Here's how the part is built. I have some questions about the finished solid (model axes, mm). Face numbers are marked on the shaded views. A direction names the side the tool comes from. Round coordinates to 2 decimals unless told otherwise and drop trailing zeros. Loops run counter-clockwise (first coordinate to the right, second up) from the corner with the lowest first, then second, coordinate; pieces in that order, holes last. Notation, with made-up numbers: M -22.5,-34 L 4.5,-34 A27 cw 4.5,-12 Z; hole C 67,-9 d6. An arc over 180 degrees is marked long. Answer as a JSON object with one key per item and string values.
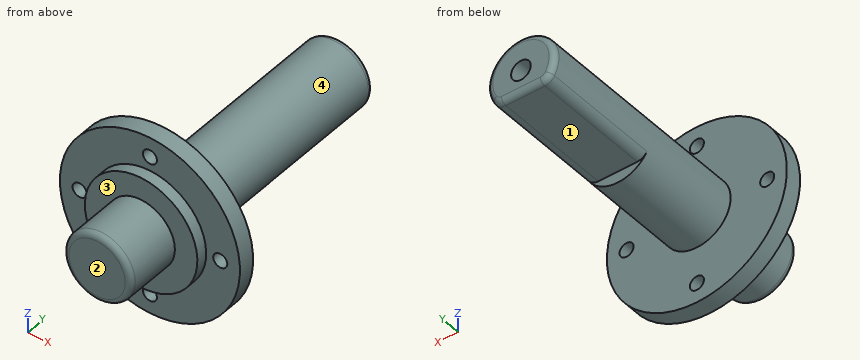
from build123d import *

# Parameters (mm, degrees)
SKETCH1_R           = 6
BOSS_EXTRUDE1_DEPTH = 10
SKETCH2_R           = 10
BOSS_EXTRUDE2_DEPTH = 2
SKETCH5_R           = 16
BOSS_EXTRUDE3_DEPTH = 3
SKETCH6_R           = 6
BOSS_EXTRUDE4_DEPTH = 40
FILLET1_R           = 1
CUT_EXTRUDE1_START  = -22
CUT_EXTRUDE1_DEPTH  = 22
FILLET2_R           = 2
FILLET3_R           = 1
SKETCH10_R          = 1.75
CUT_EXTRUDE2_DEPTH  = 20
SKETCH11_R          = 1.25
CUT_EXTRUDE3_DEPTH  = 7


with BuildPart() as part:
    # Sketch1 → Boss-Extrude1 (new body)
    with BuildSketch(Plane(origin=(0, 0, 0), x_dir=(1, 0, 0), z_dir=(0, 1, 0))):
        with Locations(Location((0, 0, 0), (0, 0, 270))):
            Circle(SKETCH1_R)
    extrude(amount=BOSS_EXTRUDE1_DEPTH)

    # Sketch2 → Boss-Extrude2 (add)
    with BuildSketch(Plane(origin=(0, 10, 0), x_dir=(1, 0, 0), z_dir=(0, 1, 0))):
        with Locations(Location((0, 0, 0), (0, 0, 270))):
            Circle(SKETCH2_R)
    extrude(amount=BOSS_EXTRUDE2_DEPTH)

    # Sketch5 → Boss-Extrude3 (add)
    with BuildSketch(Plane(origin=(0, 12, 0), x_dir=(1, 0, 0), z_dir=(0, 1, 0))):
        with Locations(Location((0, 0, 0), (0, 0, 270))):
            Circle(SKETCH5_R)
    extrude(amount=BOSS_EXTRUDE3_DEPTH)

    # Sketch6 → Boss-Extrude4 (add)
    with BuildSketch(Plane(origin=(0, 15, 0), x_dir=(1, 0, 0), z_dir=(0, 1, 0))):
        with Locations(Location((0, 0, 0), (0, 0, 270))):
            Circle(SKETCH6_R)
    extrude(amount=BOSS_EXTRUDE4_DEPTH)

    # Fillet1
    fillet1_edges = [part.edges().sort_by_distance(p)[0] for p in [
        (0, 0, -6),
    ]]
    fillet(fillet1_edges, radius=FILLET1_R)

    # Sketch7 → Cut-Extrude1 (cut)
    with BuildSketch(Plane(origin=(0, 55, 0), x_dir=(1, 0, 0), z_dir=(0, 1, 0)).offset(CUT_EXTRUDE1_START)):
        with BuildLine():
            Line((-4.472135955, 4), (4.472135955, 4))
            ThreePointArc((4.472135955, 4), (0, 6), (-4.472135955, 4))
        make_face()
    extrude(amount=CUT_EXTRUDE1_DEPTH, mode=Mode.SUBTRACT)

    # Fillet2
    fillet2_edges = [part.edges().sort_by_distance(p)[0] for p in [
        (-4.472135955, 44, -4),
        (4.472135955, 44, -4),
    ]]
    fillet(fillet2_edges, radius=FILLET2_R)

    # Fillet3
    fillet3_edges = [part.edges().sort_by_distance(p)[0] for p in [
        (5.196152423, 55, 3),
        (0, 55, -4),
        (-4.464101615, 55, -3.732050808),
        (4.464101615, 55, -3.732050808),
    ]]
    fillet(fillet3_edges, radius=FILLET3_R)

    # Sketch10 → Cut-Extrude2 (cut)
    with BuildSketch(Plane(origin=(0, 55, 0), x_dir=(1, 0, 0), z_dir=(0, 1, 0))):
        with Locations(Location((0, 0, 0), (0, 0, 270))):
            Circle(SKETCH10_R)
    extrude(amount=-CUT_EXTRUDE2_DEPTH, mode=Mode.SUBTRACT)

    # Sketch11 → Cut-Extrude3 (cut)
    with BuildSketch(Plane(origin=(0, 15, 0), x_dir=(1, 0, 0), z_dir=(0, 1, 0))):
        with Locations(Location((0, 12.5, 0), (0, 0, 270))):
            Circle(SKETCH11_R)
        with Locations(Location((12.5, 0, 0), (0, 0, 270))):
            Circle(SKETCH11_R)
        with Locations(Location((0, -12.5, 0), (0, 0, 270))):
            Circle(SKETCH11_R)
        with Locations(Location((-12.5, 0, 0), (0, 0, 270))):
            Circle(SKETCH11_R)
    extrude(amount=-CUT_EXTRUDE3_DEPTH, mode=Mode.SUBTRACT)


solid = part.part
Item 1: On a 3-axis mill with a long thin cutter (end or side, diameter ignored), from which of +Z, -Z, +X, -X, +Y, -Y can I reach the whole of each face in a straight line? I mean the marked faces 1, 2, 3 and 4. Say none if no direction works.
Resolved:
{"face 1": "-Z, +X, -X, +Y", "face 2": "+Z, -Z, +X, -X, -Y", "face 3": "-Y", "face 4": "+Y"}
Item 2: I want a section at A-A, the plane z = 12.5. Please give me the cut outline in (x, y), then the cut area to 3 significant figures.
Resolved:
{"outline": "M -9.99,12 L -1.25,12 L -1.25,15 L -9.99,15 Z; M 1.25,12 L 9.99,12 L 9.99,15 L 1.25,15 Z", "area": "52.4 mm²"}
Item 3: I want a section at D-D, the plane y = 50. Please give me the cut outline in (x, z), then the cut area to 3 significant figures.
Resolved:
{"outline": "M -5.2,-3 A2 ccw -3.46,-4 L 3.46,-4 A2 ccw 5.2,-3 A6 ccw long Z; hole C 0,0 d3.5", "area": "90.8 mm²"}
Item 4: I want a section at C-C, the plane x = 0. State how many separate pieces and enclosed holes the cut face has, then the cut area to 3 significant figures.
Resolved:
{"separate pieces": "3", "enclosed holes": "0", "area": "606 mm²"}
Item 5: I want a section at B-B, the plane x = 12.5. Please give me the cut outline in (y, z), then the cut area to 3 significant figures.
Resolved:
{"outline": "M 12,-9.99 L 15,-9.99 L 15,-1.25 L 12,-1.25 Z; M 12,1.25 L 15,1.25 L 15,9.99 L 12,9.99 Z", "area": "52.4 mm²"}
Item 6: I'm going to push flat-ended pins straight in: pin 1 Ø3 at (x, z) = (0, 0) entering from -Y; pin 2 Ø1.5 at (x, z) = (11, 3.5) entering from +Y; pin 3 Ø2 at (x, z) = (-12.5, 0) entering from +Y; pin 4 Ø1.5 at (x, y) = (3.5, 34) entering from -Z. Where does each tip first touch, or does it pass through?
Resolved:
{"pin 1": "y = 0", "pin 2": "y = 15", "pin 3": "through", "pin 4": "z = -4"}
Item 7: Please list where these lines run through material, in increasing order: probe 1 along X at (y, z) = (13.4, 0); probe 2 along Y at (x, z) = (5, 1); probe 3 along Y at (x, z) = (-2, 14). Write a range as from..to.
Resolved:
{"probe 1": "-16..-13.75, -11.25..11.25, 13.75..16", "probe 2": "0..55", "probe 3": "12..15"}
